Verification items for the finished model (mm, model axes). A direction names the side the tool comes from. Coordinates: 2 decimals unless noted, no trailing zeros. Loops run counter-clockwise (first coordinate to the right, second up) from the corner with the lowest first, then second, coordinate; pieces in that order, holes last. Notation, with made-up numbers: (35.5, -37.75) -> (91.5, -37.75) arc R9 ccw to (91.5, -31.75) -> close; hole circle Ø5 at (75, 54). An arc over 180 degrees is marked (long way). Answer as a JSON object with one key per item and string values. Group by question number.
Q1. Set-up check for faces 1 (the cylindrical face through (54.28, -57.81, -3.3)), 2 (the cylindrical face through (55.22, -43.66, 0.49)), 3 (the cylindrical face through (50.867, -57.806, -4.715)): record each of +Z, -Z, +X, -X, +Y, -Y from which the full face is reachable in a straight line by a thin tool's end or side.
Q2. Cross-section at B-B on x = 55.25. Record the boundary of the cut face in (y, z).
Q3. Gauge pin test, flat ends, axial feed: pin 1 Ø0.7 at (y, z) = (-37, -1) entering from +X; pin 2 Ø3 at (y, z) = (-40, 0) entering from +X; pin 3 Ø5 at (x, y) = (57.5, -53.5) entering from -Z. Record the tip position at first contact, or that the pin passes through.
Q4. Cross-section at C-C on x = 54. Record the boundary of the cut face in (y, z).
Q5. Release check for a two-part mould opening along Y. For faces 4 (the cylindrical face through (59.68, -58.446, 0.493)), 5 (the flat face through (52, -36.411, -1)), 6 (the flat face through (53, -48, 0)), 7 (the flat face through (53, -38, -5)) record: released by +Y, released by -Y, zero draft, split by the parting line, or undercut.
Q6. Cross-section at D-D on x = 52.5. Record the boundary of the cut face in (y, z), and give its area (3 significant figures).
Q7. Scan lines: L1, parallel to Y at x = 51, z = -0.75; L2, parallel to Z at x = 51, y = -46.25; L3, parallel to X at y = -38.25, z = -1. Record each from-to range of solid material in increasing order.
Q8. Cross-section at A-A on z = -1.75. Record the boundary of the cut face in (x, y), and give its area (3 significant figures).
```python
from build123d import *

# Parameters (mm, degrees)
BOSS_EXTRUDE1_DEPTH  = 1
FILLET1_START        = -1
FILLET1_DEPTH        = 3
FILLET2_START        = -1
FILLET2_DEPTH        = 3
SKETCH2_W            = 2.148941634
SKETCH2_H            = 2.454875289
BOSS_EXTRUDE2_DEPTH  = 4
SKETCH3_W            = 4
SKETCH3_H            = 2.454875289
BOSS_EXTRUDE3_DEPTH  = 2
FILLET3_R            = 1
FILLET3_OF_MIRROR1_R = 1
FILLET4_R            = 2


with BuildPart() as part:
    # Sketch1 → Boss-Extrude1 (new body)
    with BuildSketch(Plane.XY):
        with BuildLine():
            Line((50.566235294, -36.41094824), (50.566235294, -59.015823529))
            Line((50.566235294, -59.015823529), (60.281235294, -59.015823529))
            Line((60.281235294, -59.015823529), (60.281235294, -54.188823529))
            ThreePointArc((60.281235294, -54.188823529), (53.781235294, -47.688823529), (60.281235294, -41.188823529))
            Line((60.281235294, -41.188823529), (60.281235294, -36.41094824))
            Line((60.281235294, -36.41094824), (50.566235294, -36.41094824))
        make_face()
    boss_extrude1 = extrude(amount=BOSS_EXTRUDE1_DEPTH)

    # Fillet1: read off the stored shape, not the designer's step
    # Fillet1 outline → Fillet1 (cut)
    with BuildSketch(Plane.XY.offset(FILLET1_START)):
        with BuildLine():
            ThreePointArc((60.281235294, -54.188823529), (59.341877232, -54.12058895), (58.422241232, -53.917317816))
            add(Edge.make_bspline(
                [(58.422241232, -53.917317816), (59.442487987, -54.221826831), (60.281235188, -55.09507753), (60.281235294, -56.412193512)],
                knots=[0, 0, 0, 0, 0.45799037, 0.45799037, 0.45799037, 0.45799037], degree=3, weights=[1, 0.738797902, 0.597223849, 0.575277842]))
            Line((60.281235294, -56.412193512), (60.281235294, -54.188823529))
        make_face()
        with BuildLine():
            Line((60.281235294, -59.015823529), (60.281235294, -56.412193512))
            add(Edge.make_bspline(
                [(60.281235294, -56.412193512), (60.28123543, -58.106912276), (59.025045045, -59.01582353), (57.677605485, -59.015823529)],
                knots=[0.45799037, 0.45799037, 0.45799037, 0.45799037, 1, 1, 1, 1], degree=3, weights=[0.575277842, 0.549305795, 0.690879848, 1]))
            Line((57.677605485, -59.015823529), (60.281235294, -59.015823529))
        make_face()
    extrude(amount=FILLET1_DEPTH, mode=Mode.SUBTRACT)

    # Fillet2: read off the stored shape, not the designer's step
    # Fillet2 outline → Fillet2 (cut)
    with BuildSketch(Plane.XY.offset(FILLET2_START)):
        with BuildLine():
            Line((60.281235294, -36.41094824), (57.705740699, -36.41094824))
            add(Edge.make_bspline(
                [(57.705740699, -36.41094824), (59.038271524, -36.41094824), (60.281235294, -37.309720888), (60.281235294, -38.986442835)],
                knots=[0, 0, 0, 0, 0.541625397, 0.541625397, 0.541625397, 0.541625397], degree=3, weights=[1, 0.690686422, 0.548904933, 0.574655534]))
            Line((60.281235294, -38.986442835), (60.281235294, -36.41094824))
        make_face()
        with BuildLine():
            Line((60.281235294, -41.188823529), (60.281235294, -38.986442835))
            add(Edge.make_bspline(
                [(60.281235294, -38.986442835), (60.281235295, -40.292334143), (59.448338906, -41.156634612), (58.436628954, -41.456053082)],
                knots=[0.541625397, 0.541625397, 0.541625397, 0.541625397, 1, 1, 1, 1], degree=3, weights=[0.574655534, 0.596448126, 0.738229615, 1]))
            ThreePointArc((58.436628954, -41.456053082), (59.349303941, -41.255977817), (60.281235294, -41.188823529))
        make_face()
    extrude(amount=FILLET2_DEPTH, mode=Mode.SUBTRACT)

    # Sketch2 → Boss-Extrude2 (add)
    with BuildSketch(Plane.XY.offset(1)):
        with Locations((51.640706111, -37.638385885)):
            Rectangle(SKETCH2_W, SKETCH2_H)
    boss_extrude2 = extrude(amount=-BOSS_EXTRUDE2_DEPTH)

    # Sketch3 → Boss-Extrude3 (add)
    with BuildSketch(Plane(origin=(0, 0, -3), x_dir=(-1, 0, 0), z_dir=(0, 0, -1))):
        with Locations((-52.566235294, -37.638385885)):
            Rectangle(SKETCH3_W, SKETCH3_H)
    boss_extrude3 = extrude(amount=BOSS_EXTRUDE3_DEPTH)

    # Fillet3
    fillet3_edges = [part.edges().sort_by_distance(p)[0] for p in [
        (54.566235294, -37.638385885, -3),
        (54.566235294, -37.638385885, -5),
        (50.566235294, -37.638385885, -5),
    ]]
    fillet(fillet3_edges, radius=FILLET3_R - 0.0001)  # a hair under: the kernel refuses the full size

    # Mirror1: Boss-Extrude1, Boss-Extrude2, Boss-Extrude3 across plane
    add(boss_extrude1.mirror(Plane.ZX.offset(-47.713385885)))
    add(boss_extrude2.mirror(Plane.ZX.offset(-47.713385885)))
    add(boss_extrude3.mirror(Plane.ZX.offset(-47.713385885)))

    # Fillet3 of Mirror1
    fillet3_of_mirror1_edges = [part.edges().sort_by_distance(p)[0] for p in [
        (54.566235294, -57.788385885, -3),
        (54.566235294, -57.788385885, -5),
        (50.566235294, -57.788385885, -5),
    ]]
    fillet(fillet3_of_mirror1_edges, radius=FILLET3_OF_MIRROR1_R - 0.0001)  # a hair under: the kernel refuses the full size

    # Fillet4
    # the kernel refuses this fillet: 2 mm, written as the material it takes off along each edge
    with BuildSketch(Plane(origin=(60.281235294, -41.23794824, -4.403389552), x_dir=(0, 1, 0), z_dir=(0, 0, 1))) as fillet4_piece_1:
        with BuildLine():
            CenterArc((1.761355821, 2), FILLET4_R, 193.608960631, 76.391039369)
            Line((-0.182492608, 1.529411765), (-0.221369576, 1.52))
            ThreePointArc((-0.221369576, 1.52), (-0.085502649, 0.765391227), (-0.04, 0))
            Line((-0.04, 0), (0, -0.04))
            Line((0, -0.04), (1.761355821, -0.04))
            Line((1.761355821, -0.04), (1.761355821, 0))
        make_face()
    extrude(amount=9.806779105, mode=Mode.SUBTRACT)
    with BuildSketch(Plane(origin=(60.281235294, -36.41094824, -5), x_dir=(-1, 0, 0), z_dir=(0, 0, 1))) as fillet4_piece_2:
        with BuildLine():
            CenterArc((FILLET4_R, FILLET4_R), FILLET4_R, 180, 90)
            Line((0, FILLET4_R), (-FILLET4_R * 0.02, FILLET4_R))
            Line((-FILLET4_R * 0.02, FILLET4_R), (-FILLET4_R * 0.02, -FILLET4_R * 0.02))
            Line((-FILLET4_R * 0.02, -FILLET4_R * 0.02), (FILLET4_R, -FILLET4_R * 0.02))
            Line((FILLET4_R, -FILLET4_R * 0.02), (FILLET4_R, 0))
        make_face()
    extrude(amount=11, mode=Mode.SUBTRACT)
    with BuildSketch(Plane(origin=(60.281235294, -59.015823529, -5), x_dir=(-1, 0, 0), z_dir=(0, 0, 1))) as fillet4_piece_3:
        with BuildLine():
            CenterArc((FILLET4_R, -FILLET4_R), FILLET4_R, 90, 90)
            Line((0, -FILLET4_R), (-FILLET4_R * 0.02, -FILLET4_R))
            Line((-FILLET4_R * 0.02, -FILLET4_R), (-FILLET4_R * 0.02, FILLET4_R * 0.02))
            Line((-FILLET4_R * 0.02, FILLET4_R * 0.02), (FILLET4_R, FILLET4_R * 0.02))
            Line((FILLET4_R, FILLET4_R * 0.02), (FILLET4_R, 0))
        make_face()
    extrude(amount=11, mode=Mode.SUBTRACT)
    with BuildSketch(Plane(origin=(60.281235294, -54.23794824, -4.399691242), x_dir=(0, -1, 0), z_dir=(0, 0, 1))) as fillet4_piece_4:
        with BuildLine():
            CenterArc((1.759876497, -2), FILLET4_R, 90, 74.48871178)
            Line((-0.167279071, -1.465143556), (-0.205822183, -1.454446427))
            ThreePointArc((-0.205822183, -1.454446427), (-0.081696985, -0.732793564), (-0.04, 0))
            Line((-0.04, 0), (0, 0.04))
            Line((0, 0.04), (1.759876497, 0.04))
            Line((1.759876497, 0.04), (1.759876497, 0))
        make_face()
    extrude(amount=9.799382485, mode=Mode.SUBTRACT)


solid = part.part
```
Computed values:
{
 "1": {"face 1": "+X, +Y, -Y", "face 2": "+Z, -Z, +X", "face 3": "-Z, -X, +Y, -Y"},
 "2": {"outline": "(-59.02, 0) -> (-51.8, 0) -> (-51.8, 1) -> (-59.02, 1) -> close; (-43.62, 0) -> (-36.41, 0) -> (-36.41, 1) -> (-43.62, 1) -> close"},
 "3": {"pin 1": "stops at x = 52.72", "pin 2": "stops at x = 60.28", "pin 3": "stops at z = 0"},
 "4": {"outline": "(-59.02, -4.9) -> (-56.56, -4.9) -> (-56.56, -3.1) -> (-59.02, -3.1) -> close; (-59.02, 0) -> (-49.36, 0) -> (-49.36, 1) -> (-59.02, 1) -> close; (-46.07, 0) -> (-36.41, 0) -> (-36.41, 1) -> (-46.07, 1) -> close; (-38.87, -4.9) -> (-36.41, -4.9) -> (-36.41, -3.1) -> (-38.87, -3.1) -> close"},
 "5": {"face 4": "released by -Y", "face 5": "released by +Y", "face 6": "undercut", "face 7": "zero draft"},
 "6": {"outline": "(-59.02, -5) -> (-56.56, -5) -> (-56.56, 0) -> (-38.87, 0) -> (-38.87, -5) -> (-36.41, -5) -> (-36.41, 1) -> (-59.02, 1) -> close", "area": "47.2 mm²"},
 "7": {"L1": "y = -59.02 to -56.56, -38.87 to -36.41", "L2": "z = 0 to 1", "L3": "x = 50.57 to 52.72"},
 "8": {"outline": "(50.57, -59.02) -> (52.72, -59.02) -> (52.72, -56.56) -> (50.57, -56.56) -> close; (50.57, -38.87) -> (52.72, -38.87) -> (52.72, -36.41) -> (50.57, -36.41) -> close", "area": "10.6 mm²"}
}
